```python
from build123d import *

# Parameters (mm, degrees)
SZKIC1_W                    = 145
SZKIC1_H                    = 182
DODANIE_WYCI_GNI_CIE1_DEPTH = 2
SZKIC2_R                    = 2
WYTNIJ_WYCI_GNI_CIE1_DEPTH  = 32
SZKIC3_W                    = 5.5
SZKIC3_H                    = 6.4
WYTNIJ_WYCI_GNI_CIE2_DEPTH  = 32
SZKIC4_R                    = 2
WYTNIJ_WYCI_GNI_CIE3_DEPTH  = 12


with BuildPart() as part:
    # Szkic1 → Dodanie-wyciągnięcie1 (new body)
    with BuildSketch(Plane.XY):
        Rectangle(SZKIC1_W, SZKIC1_H)
    extrude(amount=DODANIE_WYCI_GNI_CIE1_DEPTH)

    # Szkic2 → Wytnij-wyciągnięcie1 (cut)
    with BuildSketch(Plane(origin=(0, 0, 0), x_dir=(-1, 0, 0), z_dir=(0, 0, -1))):
        with Locations((-22.5, -11)):
            Circle(SZKIC2_R)
        with Locations((-22.5, -71)):
            Circle(SZKIC2_R)
        with Locations((22.5, -71)):
            Circle(SZKIC2_R)
        with Locations((22.5, -11)):
            Circle(SZKIC2_R)
    extrude(amount=-WYTNIJ_WYCI_GNI_CIE1_DEPTH, mode=Mode.SUBTRACT)

    # Szkic3 → Wytnij-wyciągnięcie2 (cut)
    with BuildSketch(Plane(origin=(0, 0, 0), x_dir=(-1, 0, 0), z_dir=(0, 0, -1))):
        with Locations((-15.6, 84.25)):
            Rectangle(SZKIC3_W, SZKIC3_H)
        with Locations((29.4, 84.25)):
            Rectangle(SZKIC3_W, SZKIC3_H)
        with Locations((-60.6, 84.25)):
            Rectangle(SZKIC3_W, SZKIC3_H)
    extrude(amount=-WYTNIJ_WYCI_GNI_CIE2_DEPTH, mode=Mode.SUBTRACT)

    # Szkic4 → Wytnij-wyciągnięcie3 (cut)
    with BuildSketch(Plane(origin=(0, 0, 0), x_dir=(-1, 0, 0), z_dir=(0, 0, -1))):
        with Locations((67.5, -86.5)):
            Circle(SZKIC4_R)
        with Locations((-67.5, -86.5)):
            Circle(SZKIC4_R)
        with Locations((-67.5, 58.5)):
            Circle(SZKIC4_R)
        with Locations((67.878744236, 58.5)):
            Circle(SZKIC4_R)
    extrude(amount=-WYTNIJ_WYCI_GNI_CIE3_DEPTH, mode=Mode.SUBTRACT)


solid = part.part
```
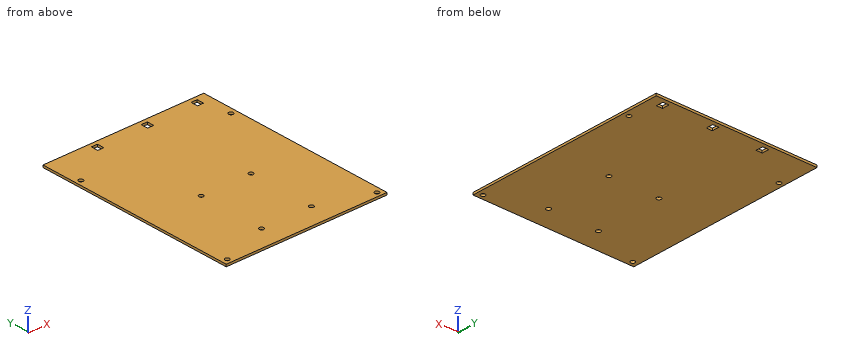
The model under review builds one solid part; all positions refer to its coordinate system, in mm. Coordinates: 2 decimals unless noted, no trailing zeros. Write each loop counter-clockwise with the first axis right and the second up, starting at its lowest first coordinate (ties: lowest second). Pieces come first, ordered by that corner, then holes. Notation, with made-up numbers: (25, 1) - (47, 1) arc R10 cw to (47, 13) - close; hole circle Ø4 at (17, 55). An arc over 180 degrees is marked (long way). Answer in a Markdown table with one row per item. Add a question column.
Q1. Consider section C-C on x = 61. Give the boundary of the cut face in (y, z), then the cut area to 3 significant figures.
Q2. To check wall thickness, follow line 1 along Y through (x, z) = (67.5, 1.45); line 2 along Y through (x, z) = (22.5, 0.45); line 3 along X through (y, z) = (-71.5, 1.7). State the ranges of each line that lie inside material, in increasing order. Write a range as from..to.
Q3. Consider section B-B on y = -86.5. Give the boundary of the cut face in (x, z), then the cut area to 3 significant figures.
Q4. Consider section A-A on x = -22.5. Give the boundary of the cut face in (y, z).
Answers below:
| question | item | result |
|---|---|---|
| 1 | outline | (-91, 0) - (81.05, 0) - (81.05, 2) - (-91, 2) - close; (87.45, 0) - (91, 0) - (91, 2) - (87.45, 2) - close |
| 1 | area | 351 mm² |
| 2 | line 1 | -91..-88.5, -84.5..56.5, 60.5..91 |
| 2 | line 2 | -91..-73, -69..-13, -9..91 |
| 2 | line 3 | -72.5..-24.44, -20.56..20.56, 24.44..72.5 |
| 3 | outline | (-72.5, 0) - (-69.5, 0) - (-69.5, 2) - (-72.5, 2) - close; (-65.5, 0) - (65.5, 0) - (65.5, 2) - (-65.5, 2) - close; (69.5, 0) - (72.5, 0) - (72.5, 2) - (69.5, 2) - close |
| 3 | area | 274 mm² |
| 4 | outline | (-91, 0) - (-73, 0) - (-73, 2) - (-91, 2) - close; (-69, 0) - (-13, 0) - (-13, 2) - (-69, 2) - close; (-9, 0) - (91, 0) - (91, 2) - (-9, 2) - close |
